Drawing for the job (mm, zero at the part's lowest x, y, z). A direction names the side the tool comes from. Give positions to 0.01 mm unless a question says otherwise; leave off trailing zeros. Loops run counter-clockwise (first coordinate to the right, second up) from the corner with the lowest first, then second, coordinate; pieces in that order, holes last.
1) 3-axis set-ups, long thin cutter, end or side, ignore diameter. For the marked faces 1 and 2: which of +Z, -Z, +X, -X, +Y, -Y reach the whole face in a straight line?
2) Band-saw the part on D-D on y = 5.5. List the corners of the cut face in (x, z), then the cut area to 3 significant figures.
3) Band-saw the part on A-A on x = 9. List the corners of the cut face in (y, z), then the cut area to 3 significant figures.
4) Band-saw the part on C-C on y = 3.5. List the corners of the cut face in (x, z), then the cut area to 3 significant figures.
5) Band-saw the part on B-B on z = 17.9. List the corners of the cut face in (x, y).
6) Two-plate mould, pull along Y, no slides. Class the marked faces 3, 4, 5 and 6: +Y half, -Y half, draft (parallel to the pull), parting line (faces both ways), or undercut.
7) Wall check: line 1 (Z direction, x = 8.7, y = 3.5); line 2 (Y direction, x = 9.45, z = 17.9); line 3 (X direction, y = 6.25, z = 10.75). Give the ranges that are in metal, low to high.
8) Flat gauge pins, fed straight in: P1, Ø6, axis at x = 3.5, z = 9.5, coming from the -Y side; P2, Ø3.5, axis at y = 3.5, z = 15.5, coming from the -X side; P3, Ø2, axis at x = 4, y = 4, coming from the +Z side. Where does each tip first touch, or does it go through?
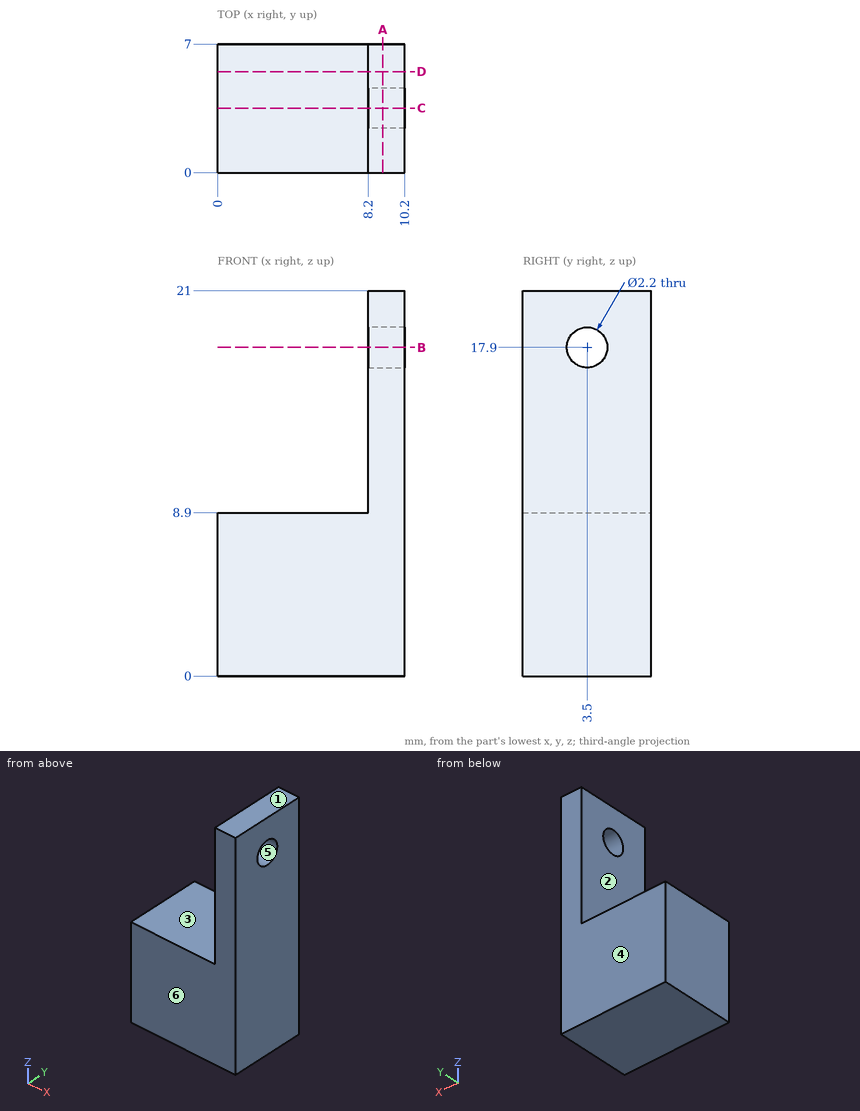
Findings below:
1. face 1: +Z, +X, -X, +Y, -Y
1. face 2: +Z, -X, +Y, -Y
2. outline: (0, 0) - (10.2, 0) - (10.2, 21) - (8.2, 21) - (8.2, 8.9) - (0, 8.9) - close
2. area: 115 mm2
3. outline: (0, 0) - (7, 0) - (7, 21) - (0, 21) - close; hole circle Ø2.2 at (3.5, 17.9)
3. area: 143 mm2
4. outline: (0, 0) - (10.2, 0) - (10.2, 16.8) - (8.2, 16.8) - (8.2, 8.9) - (0, 8.9) - close; (8.2, 19) - (10.2, 19) - (10.2, 21) - (8.2, 21) - close
4. area: 111 mm2
5. outline: (8.2, 0) - (10.2, 0) - (10.2, 2.4) - (8.2, 2.4) - close; (8.2, 4.6) - (10.2, 4.6) - (10.2, 7) - (8.2, 7) - close
6. face 3: draft
6. face 4: +Y half
6. face 5: undercut
6. face 6: -Y half
7. line 1: z = 0 to 16.8, 19 to 21
7. line 2: y = 0 to 2.4, 4.6 to 7
7. line 3: x = 8.2 to 10.2
8. P1: stops at y = 0
8. P2: stops at x = 8.2
8. P3: stops at z = 8.9
